```python
from build123d import *


with BuildPart() as f2:
    # F2: sweep along a path in F1
    with BuildLine(Plane.XY) as f2_path:
        ThreePointArc((-42.775339, -92.156554), (-9.690307, -51.507719), (0, 0))
    # F0 (on Front) → F2 (sweep)
    with BuildSketch(Plane.XZ):
        with BuildLine():
            ThreePointArc((-20.63977, -29.72378), (-32.065525, -16.772159), (-36.187058, 0))
            Line((-36.187058, 0), (-36.187058, 27.704396))
            ThreePointArc((-36.187058, 27.704396), (-38.341088, 30.969492), (-41.983402, 32.395763))
            Line((-41.983402, 32.395763), (-50.8, 32.395763))
            Line((-50.8, 32.395763), (-50.8, 0))
            ThreePointArc((-50.8, 0), (-44.088108, -25.236456), (-25.726035, -43.804237))
            Line((-25.726035, -43.804237), (0, -43.804237))
            Line((0, -43.804237), (25.726035, -43.804237))
            ThreePointArc((25.726035, -43.804237), (44.088108, -25.236456), (50.8, 0))
            Line((50.8, 0), (50.8, 32.395763))
            Line((50.8, 32.395763), (41.983402, 32.395763))
            ThreePointArc((41.983402, 32.395763), (38.341088, 30.969492), (36.187058, 27.704396))
            Line((36.187058, 27.704396), (36.187058, 0))
            ThreePointArc((36.187058, 0), (32.065525, -16.772159), (20.63977, -29.72378))
            ThreePointArc((20.63977, -29.72378), (16.846551, -31.580554), (12.671795, -32.218926))
            Line((12.671795, -32.218926), (0, -32.218926))
            Line((0, -32.218926), (-12.671795, -32.218926))
            ThreePointArc((-12.671795, -32.218926), (-16.846551, -31.580554), (-20.63977, -29.72378))
        make_face()
    sweep(path=f2_path.line)


solid = f2.part
```
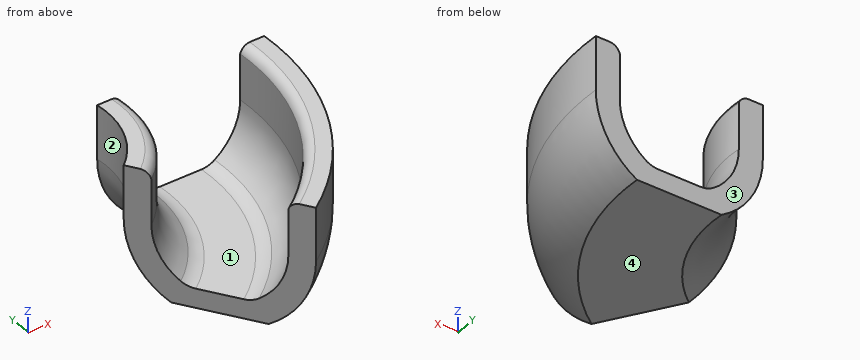
The model under review builds one solid part; all positions refer to its coordinate system, in mm. Face numbers are marked on the shaded views. Round coordinates to 2 decimals unless told otherwise and drop trailing zeros. Loops run counter-clockwise (first coordinate to the right, second up) from the corner with the lowest first, then second, coordinate; pieces in that order, holes last. Notation, with made-up numbers: (78, -36.75) -> (101, -36.75) arc R16 ccw to (101, -30.75) -> close; hole circle Ø3 at (-22, 38). An arc over 180 degrees is marked (long way). Answer in a Markdown table with one row per item.
1) Consider section A-A, the plane z = 19.5. Write out the cut boundary in (x, y).
Taken from the geometry:
| item | result |
|---|---|
| outline | (-70.46, -49.56) -> (-62.5, -61.82) arc R70.42 ccw to (-36.19, 0) -> (-50.8, 0) arc R55.89 cw to start; (-23.05, -122.5) -> (-15.09, -134.75) arc R157.24 ccw to (50.8, 0) -> (36.19, 0) arc R142.64 cw to start |
2) Draft analysis for pull direction Y (two halves, no side actions). For the marked faces 1, 2, 3 and 4, state which applies: pulls with the +Y half, pulls with the -Y half, needs draft (parallel to the pull), parting line crosses it, or undercut.
Taken from the geometry:
| item | result |
|---|---|
| face 1 | undercut |
| face 2 | undercut |
| face 3 | pulls with the +Y half |
| face 4 | needs draft |
3) For pin 1 Ø10 at (y, z) = (-20, -8.5) entering from -X; pin 2 Ø12 at (x, y) = (-53.5, -45.5) entering from -Z; pin 3 Ø3 at (x, z) = (12, 0.5) entering from -Y, all flat-tipped, find the tip position at first contact; note any pin that passes through.
Taken from the geometry:
| item | result |
|---|---|
| pin 1 | stops at x = -52.91 |
| pin 2 | stops at z = -36.75 |
| pin 3 | stops at y = -111.94 |
4) Wall thickness on line 1 along X through (y, z) = (-8, -31); line 2 along X through (y, z) = (-39.5, -16.5); line 3 along Z through (x, y) = (-4, -69.5): over which ranges is each line inside the solid? List them lowest first.
Taken from the geometry:
| item | result |
|---|---|
| line 1 | x = -39.92 to -18.14, 18.55 to 40.39 |
| line 2 | x = -57.72 to -39.54, 28.42 to 44.66 |
| line 3 | z = -43.8 to -32.19 |
